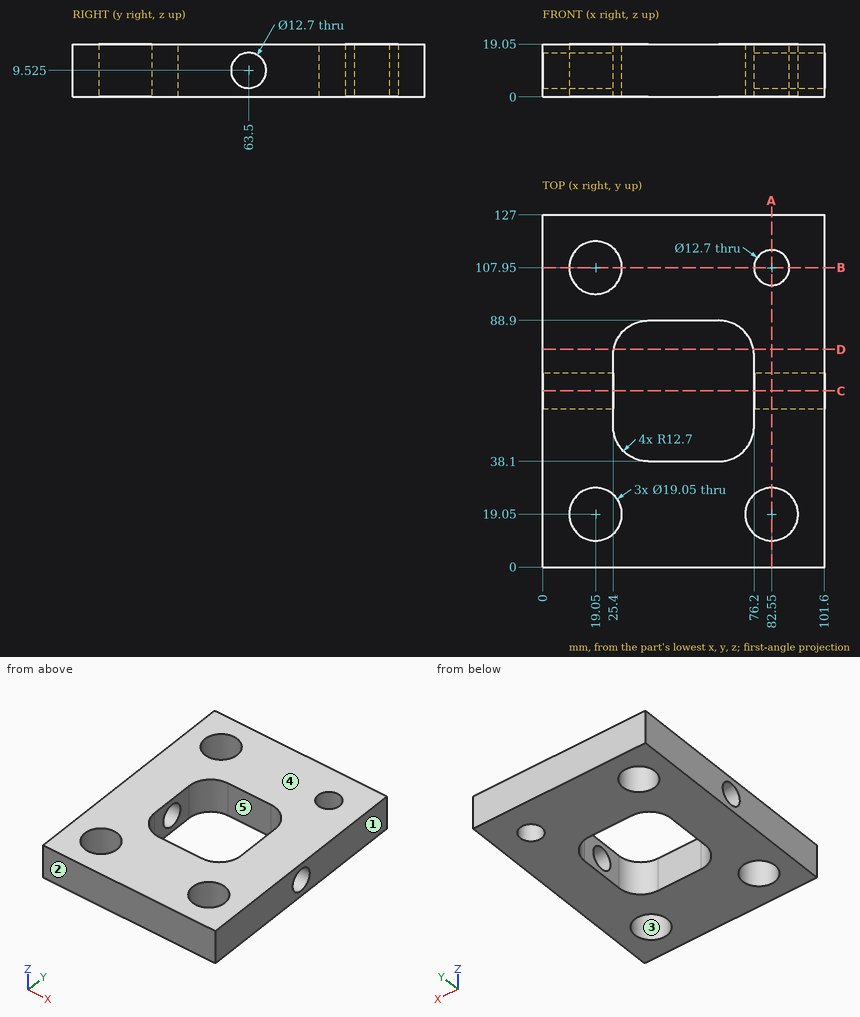
Design review of the part shown in the three views and the two pictorial views. Dimensions are in mm from the part's minimum x, y and z. A direction names the side the tool comes from. Give positions to 0.01 mm unless a question says otherwise; leave off trailing zeros. Write each loop counter-clockwise with the first axis right and the second up, starting at its lowest first coordinate (ties: lowest second). Pieces come first, ordered by that corner, then holes.
(1) Tool access review of the marked faces 4 and 5: name each direction out of +Z, -Z, +X, -X, +Y, -Y from which nothing blocks a thin tool from reaching the whole face with its end or side.
Checked values:
face 4: +Z, +X, -X, +Y, -Y
face 5: +Z, -Z
(2) Mouldability with a two-part tool opening along X and no side actions: class the marked faces 1, 2 and 3 as +X half, -X half, draft (parallel to the pull), parting line (faces both ways), or undercut.
Checked values:
face 1: +X half
face 2: draft
face 3: undercut
(3) Add section B-B (y = 107.95). Give the boundary of the cut face in (x, z) (3 decimals), and give its area (3 significant figures).
Checked values:
outline: (0, 0) - (9.525, 0) - (9.525, 19.05) - (0, 19.05) - close; (28.575, 0) - (76.2, 0) - (76.2, 19.05) - (28.575, 19.05) - close; (88.9, 0) - (101.6, 0) - (101.6, 19.05) - (88.9, 19.05) - close
area: 1,330 mm2
(4) Add section D-D (y = 78.5). Give the boundary of the cut face in (x, z).
Checked values:
outline: (0, 0) - (25.61, 0) - (25.61, 19.05) - (0, 19.05) - close; (75.99, 0) - (101.6, 0) - (101.6, 19.05) - (75.99, 19.05) - close
(5) Add section A-A (x = 82.55). Give the boundary of the cut face in (y, z) (3 decimals), and give its area (3 significant figures).
Checked values:
outline: (0, 0) - (9.525, 0) - (9.525, 19.05) - (0, 19.05) - close; (28.575, 0) - (101.6, 0) - (101.6, 19.05) - (28.575, 19.05) - close; (114.3, 0) - (127, 0) - (127, 19.05) - (114.3, 19.05) - close; hole circle Ø12.7 at (63.5, 9.525)
area: 1,690 mm2
(6) Wall thickness on line 1 along Z through (x, y) = (10.75, 63.5) (3 decimals); line 2 along Y through (x, z) = (39, 4.25); line 3 along X through (y, z) = (22, 10): over which ranges is each line inside the solid? List them lowest first.
Checked values:
line 1: z = 0 to 3.175, 15.875 to 19.05
line 2: y = 0 to 38.1, 88.9 to 127
line 3: x = 0 to 9.99, 28.11 to 73.49, 91.61 to 101.6
(7) Clearance check with a flat-ended pin moving along its axis: pin 1 Ø3 at (x, z) = (35, 15.5) entering from -Y. State where the tip first meets the part, or that it passes through.
Checked values:
pin 1: stops at y = 0
(8) Add section C-C (y = 63.5). Give the boundary of the cut face in (x, z) (3 decimals).
Checked values:
outline: (0, 0) - (25.4, 0) - (25.4, 3.175) - (0, 3.175) - close; (0, 15.875) - (25.4, 15.875) - (25.4, 19.05) - (0, 19.05) - close; (76.2, 0) - (101.6, 0) - (101.6, 3.175) - (76.2, 3.175) - close; (76.2, 15.875) - (101.6, 15.875) - (101.6, 19.05) - (76.2, 19.05) - close
